Can you work these out from the model? Positions are in its coordinate system, mm. A direction names the side the tool comes from. Round coordinates to 2 decimals unless told otherwise and drop trailing zeros. Write each loop counter-clockwise with the first axis right and the second up, starting at its lowest first coordinate (ties: lowest second). Pieces come first, ordered by that corner, then holes.
Q1. If we section it at D-D (z = 6): Please give me the cut outline in (x, y).
Q2. I'm going to push flat-ended pins straight in: pin 1 Ø1.5 at (y, z) = (-74.5, 55) entering from +X; pin 2 Ø12 at (x, z) = (-5.5, 46.5) entering from +Y; pin 3 Ø6 at (x, z) = (-1, 46) entering from +Y. Where does each tip first touch, or does it pass through?
Q3. If we section it at B-B (x = 0): Please give me the cut outline in (y, z).
Q4. Please list where these lines run through material, in increasing order: line 1 along X through (y, z) = (-61, 34); line 2 along Y through (x, z) = (-4.5, 13.5); line 3 along Z through (x, y) = (0, -74.75).
Q5. If we section it at A-A (y = -72): Please give me the cut outline in (x, z).
Q6. For faces 1 (the flat face through (-11, -60, 58)), 2 (the flat face through (-10, -55, 35)), 3 (the flat face through (-5, -74, 54)), which set-ups out of +Z, -Z, +X, -X, +Y, -Y let a thin tool reach every point of the face, with its end or its side?
Q7. We'd pull the mould along Z, two halves only. Please class faces 4 (the flat face through (11, -60, 58)), 5 (the cylindrical face through (-12.14, -74.9, 29.41)), 6 (the cylindrical face through (11.52, -35.56, 48.25)): +Z half, -Z half, draft (parallel to the pull), parting line (faces both ways), or undercut.
Q8. If we section it at C-C (z = 51): Please give me the cut outline in (x, y).
from build123d import *

# Parameters (mm, degrees)
EXTRUDE_1_DEPTH     = 58
SKETCH_2_R          = 3.25
CUT_EXTRUDE_1_DEPTH = 27
FILLET_1_R          = 7
SKETCH_3_R          = 4.5
CUT_EXTRUDE_2_DEPTH = 4
FILLET_2_R          = 3


with BuildPart() as part:
    # 草图1 → 凸台-拉伸1 (new body)
    with BuildSketch(Plane.XY):
        Polygon((-10, -20.797836643), (-10, -72.797836643), (10, -72.797836643), (10, -20.797836643), (13, -20.797836643), (13, -75.797836643), (-13, -75.797836643), (-13, -20.797836643), align=None)
    extrude(amount=EXTRUDE_1_DEPTH)

    # 草图2 → 切除-拉伸1 (cut, through all)
    with BuildSketch(Plane(origin=(13, 0, 0), x_dir=(0, 0, -1), z_dir=(1, 0, 0))):
        with Locations((-50, -38.297836643)):
            Circle(SKETCH_2_R)
        Polygon((-58, -20.797836643), (-58, -22.797836643), (0, -55.797836643), (0, -20.797836643), align=None)
    extrude(amount=-CUT_EXTRUDE_1_DEPTH, mode=Mode.SUBTRACT)

    # 圆角1
    fillet_1_edges = [part.edges().sort_by_distance(p)[0] for p in [
        (11.5, -22.797836643, 58),
        (-11.5, -22.797836643, 58),
    ]]
    fillet(fillet_1_edges, radius=FILLET_1_R)

    # 草图3 → 切除-拉伸2 (cut, through all)
    with BuildSketch(Plane(origin=(0, -72.797836643, 0), x_dir=(1, 0, 0), z_dir=(0, 1, 0))):
        with Locations((0, -12)):
            Circle(SKETCH_3_R)
        with BuildLine():
            Line((5, -49), (5, -58))
            Line((5, -58), (-5, -58))
            Line((-5, -58), (-5, -49))
            ThreePointArc((-5, -49), (0, -44), (5, -49))
        make_face()
    extrude(amount=-CUT_EXTRUDE_2_DEPTH, mode=Mode.SUBTRACT)

    # 圆角2
    fillet_2_edges = [part.edges().sort_by_distance(p)[0] for p in [
        (13, -75.797836643, 29),
        (-13, -75.797836643, 29),
    ]]
    fillet(fillet_2_edges, radius=FILLET_2_R)


solid = part.part
A:
1. outline: (-13, -72.8) arc R3 ccw to (-10, -75.8) - (10, -75.8) arc R3 ccw to (13, -72.8) - (13, -52.38) - (10, -52.38) - (10, -72.8) - (-10, -72.8) - (-10, -52.38) - (-13, -52.38) - close
2. pin 1: stops at x = 12.84
2. pin 2: stops at y = -27.85
2. pin 3: stops at y = -72.8
3. outline: (-75.8, 0) - (-72.8, 0) - (-72.8, 7.5) - (-75.8, 7.5) - close; (-75.8, 16.5) - (-72.8, 16.5) - (-72.8, 44) - (-75.8, 44) - close
4. line 1: x = -13 to -10, 10 to 13
4. line 2: y = -75.8 to -72.8
4. line 3: z = 0 to 7.5, 16.5 to 44
5. outline: (-13, 0) - (-10, 0) - (-10, 58) - (-13, 58) - close; (10, 0) - (13, 0) - (13, 58) - (10, 58) - close
6. face 1: +Z, +X, -X, +Y, -Y
6. face 2: +Z, -Z, +Y
6. face 3: +Z, +Y, -Y
7. face 4: +Z half
7. face 5: draft
7. face 6: undercut
8. outline: (-13, -72.8) arc R3 ccw to (-10, -75.8) - (-5, -75.8) - (-5, -72.8) - (-10, -72.8) - (-10, -41.39) - (-13, -41.39) - close; (-13, -35.21) - (-10, -35.21) - (-10, -27.83) - (-13, -27.83) - close; (5, -75.8) - (10, -75.8) arc R3 ccw to (13, -72.8) - (13, -41.39) - (10, -41.39) - (10, -72.8) - (5, -72.8) - close; (10, -35.21) - (13, -35.21) - (13, -27.83) - (10, -27.83) - close
